Could you check a few things on this model? Use its own coordinates, in mm. Face numbers are marked on the shaded views. A direction names the side the tool comes from. Round coordinates to 2 decimals unless told otherwise and drop trailing zeros. Put each result on its own line as item: value. Start each with the question number.
1. I need wall thicknesses on line 1 (X direction, y = 34.5, z = -51); line 2 (X direction, y = 74.5, z = -100); line 3 (Z direction, x = -66, y = 108). Which ranges of each line are inside material? Lowest first, please. Write a range as [from, to].
2. Imagine slicing it at A-A, the plane z = -12. Count the separate pieces of the cut face and the enclosed holes in it, and give its area (3 significant figures).
3. If we mould it in two halves opening along X, with no side actions, what happens to the marked faces 3, 4 and 5? For each: pulls with the +X half, pulls with the -X half, needs draft (parallel to the pull), parting line crosses it, or undercut.
4. I'm going to push flat-ended pins straight in: P1, Ø4, axis at x = 138.5, y = 31, coming from the -Z side; P2, Ø2, axis at y = 88.5, z = -30.5, coming from the +X side; P3, Ø5, axis at x = -171.5, y = 73.5, coming from the -Z side; P4, Ø9.5, axis at x = -64, z = -192.5, coming from the -Y side. Where does each tip first touch, or does it pass through?
5. Which directions (+Z, -Z, +X, -X, +Y, -Y) give clear straight access to the entire face, cutting with the end or side of a thin tool? Please do the marked faces 1 and 2.
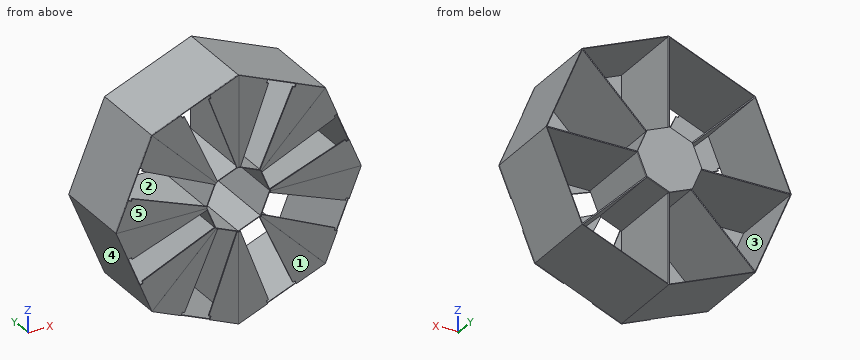
```python
from build123d import *

# Parameters (mm, degrees)
BOSS_EXTRUDE1_DEPTH = 150
BOSS_EXTRUDE2_DEPTH = 3
BOSS_EXTRUDE3_DEPTH = 2
CIRPATTERN1_COUNT   = 8


with BuildPart() as part:
    # Sketch1 → Boss-Extrude1 (new body)
    with BuildSketch(Plane(origin=(0, 0, 0), x_dir=(1, 0, 0), z_dir=(0, 1, 0))):
        Polygon((227.244412963, 0), (160.686065393, 160.686065393), (0, 227.244412963), (-160.686065393, 160.686065393), (-227.244412963, 0), (-160.686065393, -160.686065393), (0, -227.244412963), (160.686065393, -160.686065393), align=None)
        Polygon((-158.959000036, -160.319047086), (-41.038336356, -42.398383406), (-1, -58.982805339), (-1, -225.7478072), align=None, mode=Mode.SUBTRACT)
        Polygon((-225.770243704, -0.945833488), (-59.036971851, -0.945833488), (-42.452549918, -40.984169844), (-160.350777095, -158.88239702), align=None, mode=Mode.SUBTRACT)
        Polygon((1, -225.7478072), (1, -58.982805339), (41.038336356, -42.398383406), (158.959000036, -160.319047086), align=None, mode=Mode.SUBTRACT)
        Polygon((160.350777095, -158.88239702), (42.452549918, -40.984169844), (59.036971851, -0.945833488), (225.770243704, -0.945833488), align=None, mode=Mode.SUBTRACT)
        Polygon((-160.319047086, 158.959000036), (-42.452549918, 41.092502868), (-59.036971851, 1.054166512), (-225.725370696, 1.054166512), align=None, mode=Mode.SUBTRACT)
        Polygon((-41.272969491, 41.327136003), (0, 58.422959726), (41.272969491, 41.327136003), (58.368793213, 0.054166512), (41.272969491, -41.218802979), (0, -58.314626701), (-41.272969491, -41.218802979), (-58.368793213, 0.054166512), align=None, mode=Mode.SUBTRACT)
        Polygon((-1, 225.7478072), (-1, 59.091138364), (-41.038336356, 42.50671643), (-158.88239702, 160.350777095), align=None, mode=Mode.SUBTRACT)
        Polygon((225.725370696, 1.054166512), (59.036971851, 1.054166512), (42.452549918, 41.092502868), (160.319047086, 158.959000036), align=None, mode=Mode.SUBTRACT)
        Polygon((158.88239702, 160.350777095), (41.038336356, 42.50671643), (1, 59.091138364), (1, 225.7478072), align=None, mode=Mode.SUBTRACT)
    extrude(amount=BOSS_EXTRUDE1_DEPTH)

    # Sketch2 → Boss-Extrude2 (add)
    with BuildSketch(Plane(origin=(0, 150, 0), x_dir=(1, 0, 0), z_dir=(0, 1, 0))):
        Polygon((0, 59.505351926), (-42.076637864, 42.076637864), (-59.505351926, 0), (-42.076637864, -42.076637864), (0, -59.505351926), (42.076637864, -42.076637864), (59.505351926, 0), (42.076637864, 42.076637864), align=None)
    extrude(amount=BOSS_EXTRUDE2_DEPTH)

    # Sketch4 → Boss-Extrude3 (add)
    with BuildSketch(Plane.XZ):
        Polygon((-43.23156875, 39.141387058), (-178.796553997, 100.662504749), (-177.049364724, 104.512527258), (-182.861362419, 106.909146045), (-160.686065393, 160.686065393), (-42.019552833, 42.019552833), align=None)
        Polygon((-58.246475638, 2.892195211), (-197.607395503, 55.249116065), (-199.094323145, 51.291289658), (-204.898691523, 53.706327244), (-227.244412963, 0), (-59.424621501, 0), align=None)
    boss_extrude3 = extrude(amount=BOSS_EXTRUDE3_DEPTH)

    # CirPattern1: Boss-Extrude3 ×8 about axis
    cirpattern1_axis = Axis((0, 0, -0.054166512), (0, 1, 0))
    for i in range(1, CIRPATTERN1_COUNT):
        add(boss_extrude3.rotate(cirpattern1_axis, i * 360 / CIRPATTERN1_COUNT))


solid = part.part
```
Entries:
1. line 1: [-206.12, -205.04], [-52.36, -49.53], [-20.53, -17.92], [17.92, 20.53], [49.53, 52.36], [205.04, 206.12]
1. line 2: [-185.82, -184.74], [-101.36, -98.53], [-1, 1], [98.53, 101.36], [184.74, 185.82]
1. line 3: [-199.91, -198.82], [-67.47, -64.64], [-1.05, 0.95], [64.53, 67.36], [198.82, 199.91]
2. separate pieces: 3
2. enclosed holes: 0
2. area: 1,540 mm^2
3. face 3: undercut
3. face 4: pulls with the -X half
3. face 5: needs draft
4. P1: z = -170.7
4. P2: x = 215.03
4. P3: z = -140.61
4. P4: through
5. face 1: +Z, -Z, +X, -X, -Y
5. face 2: +Y
